```python
from build123d import *

# Parameters (mm, degrees)
P_IDAT_VYSUNUT_M1_DEPTH = 1.7
SKICA2_W                = 160
SKICA2_H                = 160
SKICA2_R                = 76
P_IDAT_VYSUNUT_M2_DEPTH = 15
SKICA4_W                = 160
SKICA4_H                = 160
P_IDAT_VYSUNUT_M3_DEPTH = 2


with BuildPart() as part:
    # Skica1 → Přidat vysunutím1 (new body)
    with BuildSketch(Plane.XY):
        with BuildLine():
            Line((-6.25, -75.742573893), (-6.25, -80))
            Line((-6.25, -80), (-80, -80))
            Line((-80, -80), (-80, 80))
            Line((-80, 80), (80, 80))
            Line((80, 80), (80, -80))
            Line((80, -80), (6.25, -80))
            Line((6.25, -80), (6.25, -75.742573893))
            ThreePointArc((6.25, -75.742573893), (0, 76), (-6.25, -75.742573893))
        make_face()
    extrude(amount=P_IDAT_VYSUNUT_M1_DEPTH)

    # Skica2 → Přidat vysunutím2 (add)
    with BuildSketch(Plane.XY.offset(1.7)):
        Rectangle(SKICA2_W, SKICA2_H)
        with Locations(Location((0, 0, 0), (0, 0, 265.282848868))):
            Circle(SKICA2_R, mode=Mode.SUBTRACT)
    extrude(amount=P_IDAT_VYSUNUT_M2_DEPTH)

    # Skica4 → Přidat vysunutím3 (add)
    with BuildSketch(Plane.XY.offset(16.7)):
        Rectangle(SKICA4_W, SKICA4_H)
    extrude(amount=P_IDAT_VYSUNUT_M3_DEPTH)


solid = part.part
```
Could you check a few things on this model? Use its own coordinates, in mm. A direction names the side the tool comes from. Coordinates: 2 decimals unless noted, no trailing zeros. Write each loop counter-clockwise with the first axis right and the second up, starting at its lowest first coordinate (ties: lowest second). Pieces come first, ordered by that corner, then holes. Notation, with made-up numbers: (-34.75, -3.5) -> (10.25, -3.5) arc R7 ccw to (10.25, 7.5) -> close; hole circle Ø7 at (47.5, 4.5). An arc over 180 degrees is marked (long way). One line per question, with ' | ' between items. Start each with the question number.
1. Please list where these lines run through material, in increasing order: line 1 along Y through (x, z) = (0, 9.5); line 2 along Z through (x, y) = (15, 19).
2. If we section it at A-A (z = 12.25): Please give me the cut outline in (x, y), and give its area (3 significant figures).
3. Will these pins go through, and if not, where does the flat tip stop? P1, Ø1, axis at x = 26.5, y = 2, coming from the -Z side; P2, Ø2, axis at x = 1, y = -77.5, coming from the -Z side.
4. If we section it at C-C (y = 0): Please give me the cut outline in (x, z).
5. For faces 1 (the face through (-41.13, 63.91, 8.23)), 2 (the face through (-1, 80, 9)), which set-ups out of +Z, -Z, +X, -X, +Y, -Y let a thin tool reach every point of the face, with its end or its side?
6. If we section it at B-B (x = 0): Please give me the cut outline in (y, z).
7. Thinking about a two-plate mould opening in X: for faces 3 (the face through (-80, -1, 9)), 4 (the face through (0, -78, 1.7)), 5 (the face through (-1, 1, 18.7)), 6 (the face through (-1, 1, 16.7)), which applies, pulls with the +X half, pulls with the -X half, needs draft (parallel to the pull), parting line crosses it, or undercut?
Return value:
1) line 1: y = -80 to -76, 76 to 80 | line 2: z = 16.7 to 18.7
2) outline: (-80, -80) -> (80, -80) -> (80, 80) -> (-80, 80) -> close; hole circle Ø152 at (0, 0) | area: 7,450 mm²
3) P1: stops at z = 16.7 | P2: stops at z = 1.7
4) outline: (-80, 0) -> (-76, 0) -> (-76, 16.7) -> (76, 16.7) -> (76, 0) -> (80, 0) -> (80, 18.7) -> (-80, 18.7) -> close
5) face 1: -Z | face 2: +Z, -Z, +X, -X, +Y
6) outline: (-80, 1.7) -> (-76, 1.7) -> (-76, 16.7) -> (76, 16.7) -> (76, 0) -> (80, 0) -> (80, 18.7) -> (-80, 18.7) -> close
7) face 3: pulls with the -X half | face 4: undercut | face 5: needs draft | face 6: undercut
